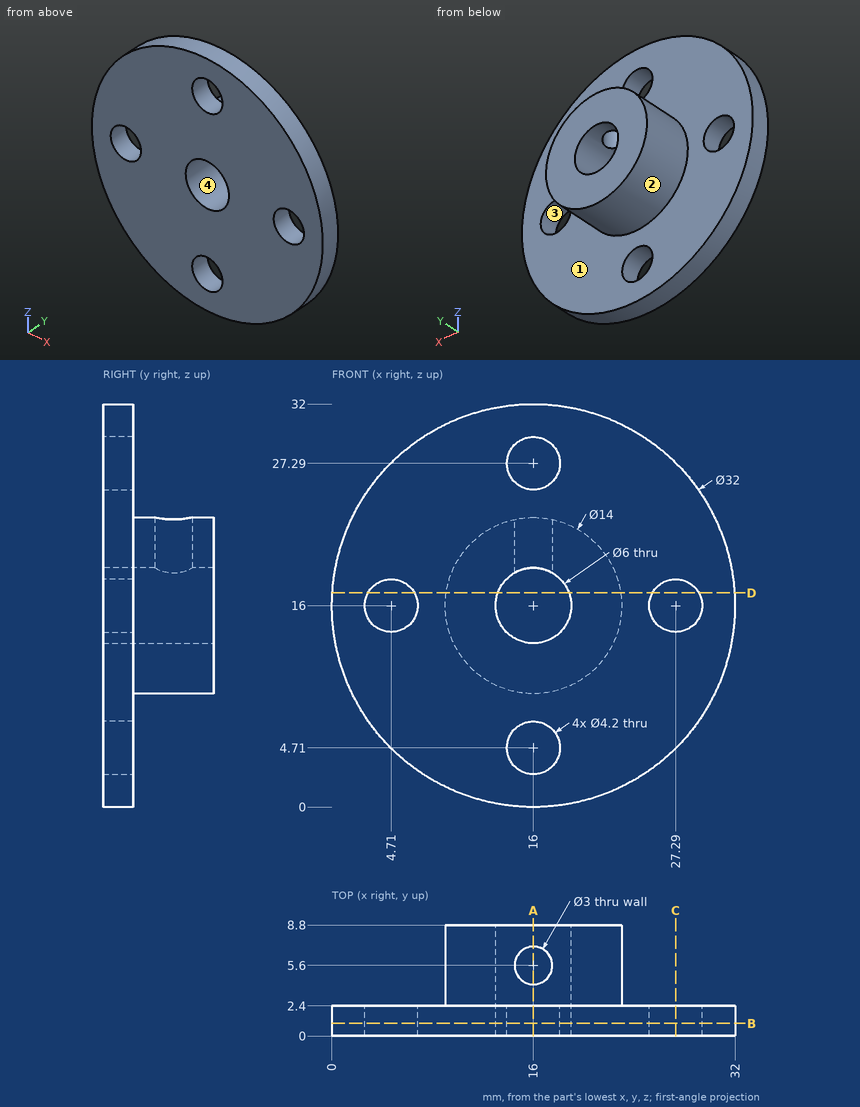
Study the drawing (mm; zero at the part's minimum x, y, z) and answer. Coordinates: 2 decimals unless noted, no trailing zeros. Loops run counter-clockwise (first coordinate to the right, second up) from the corner with the lowest first, then second, coordinate; pieces in that order, holes last. Notation, with made-up numbers: M -2.75,78.5 L 23.25,78.5 A23 ccw 23.25,108.5 Z; hole C -7,-36.5 d3. An arc over 180 degrees is marked long. Answer as a JSON object with one key per item and string values. Group by question number.
Item 1: Section C-C (x = 27.29) is taken. Write down the section's boundary in (y, z).
Item 2: Section A-A (x = 16) is taken. Write down the section's boundary in (y, z).
Item 3: Determine the mould class of the marked faces 1, 2, 3 and 4 for opening direction Z: +Z half, -Z half, draft (parallel to the pull), parting line (faces both ways), or undercut.
Item 4: Section D-D (z = 17) is taken. Write down the section's boundary in (x, y).
Item 5: Section B-B (y = 1) is taken. Write down the section's boundary in (x, z).
Item 6: Consider L1, parallel to X at y = 2, z = 16; L2, parallel to X at y = 7.25, z = 16; L3, parallel to Z at x = 16.5, y = 2.25. Determine where each line is inside the solid, lowest interval first.
Item 7: Each of these flat-tipped pins is pushed along its axis until it touches: P1, Ø1.5, axis at y = 4, z = 12, coming from the +X side; P2, Ø5.5, axis at x = 4.71, z = 16, coming from the +Y side; P3, Ø3.5, axis at x = 16, y = 5.6, coming from the -Z side; P4, Ø2.5, axis at x = 16, z = 27.29, coming from the +Y side. Where does it stop, or does it pass through?
Solved:
{
 "1": {"outline": "M 0,4.66 L 2.4,4.66 L 2.4,13.9 L 0,13.9 Z; M 0,18.1 L 2.4,18.1 L 2.4,27.34 L 0,27.34 Z"},
 "2": {"outline": "M 0,0 L 2.4,0 L 2.4,2.61 L 0,2.61 Z; M 0,6.81 L 2.4,6.81 L 2.4,9 L 8.8,9 L 8.8,13 L 0,13 Z; M 0,19 L 4.1,19 L 4.1,23 L 2.4,23 L 2.4,25.19 L 0,25.19 Z; M 0,29.39 L 2.4,29.39 L 2.4,32 L 0,32 Z; M 7.1,19 L 8.8,19 L 8.8,23 L 7.1,23 Z"},
 "3": {"face 1": "draft", "face 2": "parting line", "face 3": "undercut", "face 4": "undercut"},
 "4": {"outline": "M 0.03,0 L 2.86,0 L 2.86,2.4 L 0.03,2.4 Z; M 6.56,0 L 13.17,0 L 13.17,8.8 L 9.07,8.8 L 9.07,2.4 L 6.56,2.4 Z; M 18.83,0 L 25.44,0 L 25.44,2.4 L 22.93,2.4 L 22.93,8.8 L 18.83,8.8 Z; M 29.14,0 L 31.97,0 L 31.97,2.4 L 29.14,2.4 Z"},
 "5": {"outline": "C 16,16 d32; hole C 4.71,16 d4.2; hole C 16,16 d6; hole C 16,4.71 d4.2; hole C 16,27.29 d4.2; hole C 27.29,16 d4.2"},
 "6": {"L1": "x = 0 to 2.61, 6.81 to 13, 19 to 25.19, 29.39 to 32", "L2": "x = 9 to 13, 19 to 23", "L3": "z = 0.01 to 2.67, 6.75 to 13.04, 18.96 to 25.25, 29.33 to 31.99"},
 "7": {"P1": "stops at x = 22.2", "P2": "stops at y = 2.4", "P3": "stops at z = 9", "P4": "passes through"}
}
